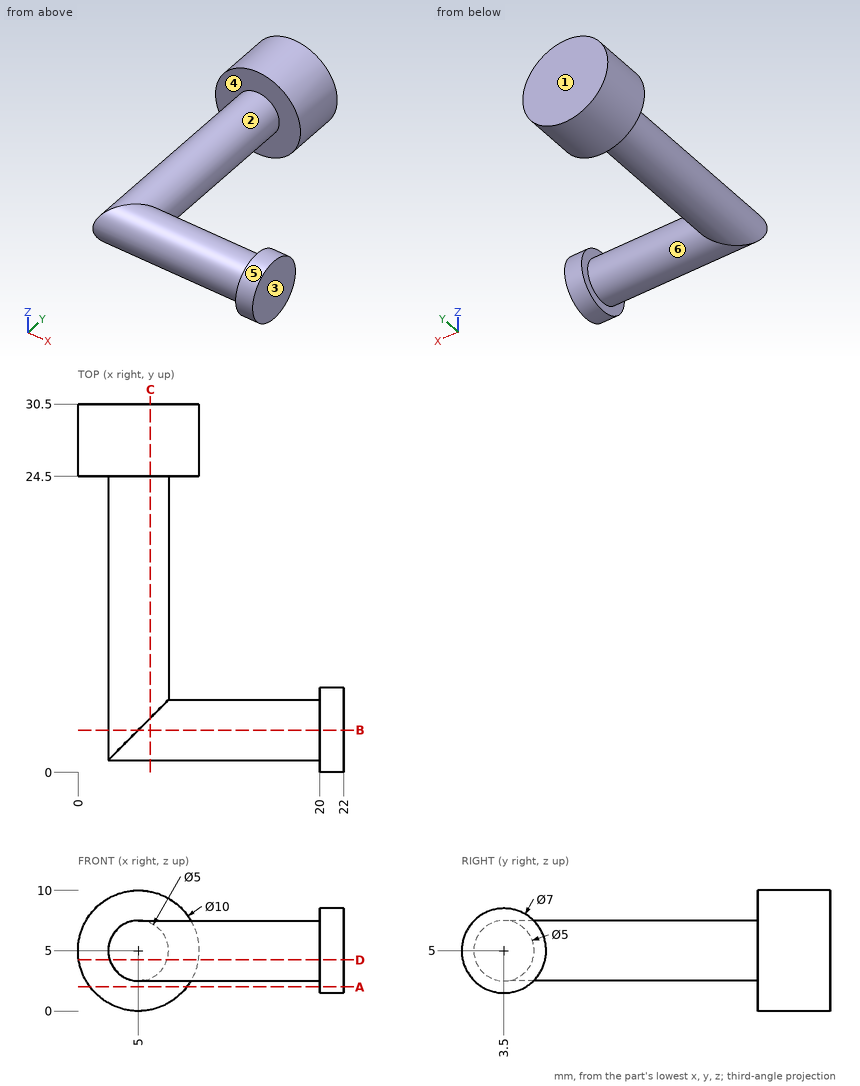
Part print with two shaded views. Sizes in mm from the minimum x, y, z corner. A direction names the side the tool comes from. Round coordinates to 2 decimals unless told otherwise and drop trailing zeros. Write each loop counter-clockwise with the first axis right and the second up, starting at its lowest first coordinate (ties: lowest second). Pieces come first, ordered by that corner, then holes. Notation, with made-up numbers: M 89,3.5 L 127,3.5 A24 cw 127,13.5 Z; hole C 88.5,-32 d11. An arc over 180 degrees is marked long. Put each result on its own line as item: value. Start each with the question number.
1) Saw through at C-C, the plane x = 6. Write the cut outline in (y, z).
2) Pin check, flat tips, straight feed: pin 1 Ø6 at (x, z) = (16, 5.5) entering from -Y; pin 2 Ø2 at (y, z) = (2.5, 4) entering from -X; pin 3 Ø4 at (y, z) = (7, 4) entering from +X; pin 4 Ø3 at (x, y) = (5, 6) entering from +Z. Stop position of each tip, or through.
3) Saw through at B-B, the plane y = 3.5. Write the cut outline in (x, z), and give its area (3 significant figures).
4) Drill centre lines: probe 1 along Y at (x, z) = (7.5, 6); probe 2 along Y at (x, z) = (2.5, 1.25); probe 3 along Y at (x, z) = (7.75, 7). Where is each one in solid material? Low to high. Write a range as [from, to].
5) Saw through at A-A, the plane z = 2. Write the cut outline in (x, y), and give its area (3 significant figures).
6) Saw through at D-D, the plane z = 4.25. Write the cut outline in (x, y), and give its area (3 significant figures).
7) Pull direction Y, two halves, no side cores. Call the marked faces 1, 2, 3 and 4: pulls with the +Y half, pulls with the -Y half, needs draft (parallel to the pull), parting line crosses it, or undercut.
8) 3-axis set-ups, long thin cutter, end or side, ignore diameter. For the marked faces 5 and 6: which of +Z, -Z, +X, -X, +Y, -Y reach the whole face in a straight line?
Resolved:
1. outline: M 4.5,2.71 L 24.5,2.71 L 24.5,0.1 L 30.5,0.1 L 30.5,9.9 L 24.5,9.9 L 24.5,7.29 L 4.5,7.29 A2.5 ccw long Z
2. pin 1: y = 1
2. pin 2: x = 2.5
2. pin 3: x = 22
2. pin 4: z = 7.5
3. outline: M 5,2.5 L 20,2.5 L 20,1.5 L 22,1.5 L 22,8.5 L 20,8.5 L 20,7.5 L 5,7.5 A2.5 ccw Z
3. area: 98.8 mm²
4. probe 1: [1.21, 5.79], [24.5, 30.5]
4. probe 2: [24.5, 30.5]
4. probe 3: [2, 5], [24.5, 30.5]
5. outline: M 1,24.5 L 9,24.5 L 9,30.5 L 1,30.5 Z; M 20,1.7 L 22,1.7 L 22,5.3 L 20,5.3 Z
5. area: 55.2 mm²
6. outline: M 0.06,24.5 L 2.62,24.5 L 2.62,1.12 L 20,1.12 L 20,0.08 L 22,0.08 L 22,6.92 L 20,6.92 L 20,5.88 L 7.38,5.88 L 7.38,24.5 L 9.94,24.5 L 9.94,30.5 L 0.06,30.5 Z
6. area: 245 mm²
7. face 1: pulls with the +Y half
7. face 2: undercut
7. face 3: needs draft
7. face 4: undercut
8. face 5: +X
8. face 6: none
